Design review of the part built by this model. Coordinates are the model's own, in mm. A direction names the side the tool comes from. Round coordinates to 2 decimals unless told otherwise and drop trailing zeros. Write each loop counter-clockwise with the first axis right and the second up, starting at its lowest first coordinate (ties: lowest second). Pieces come first, ordered by that corner, then holes. Notation, with made-up numbers: (69.5, -7) - (105.5, -7) arc R28 ccw to (105.5, 28) - close; hole circle Ø5 at (27, 11.25). An arc over 180 degrees is marked (long way). Use one line per item in the form item = value.
```python
from build123d import *

# Parameters (mm, degrees)
F1_DEPTH = 50
F2_SIZE  = 1


with BuildPart() as f1:
    # F0 (on Top) → F1 (new body)
    with BuildSketch(Plane.XY):
        Polygon((-45.5, 0), (0, 0), (0, -59.5), (-4, -59.5), (-4, -62.5), (4, -62.5), (4, 4), (-14.25, 4), (-16.5, 4), (-29, 4), (-31.25, 4), (-49.5, 4), (-49.5, -62.5), (-41.5, -62.5), (-41.5, -59.5), (-45.5, -59.5), align=None)
        Polygon((-16.5, 4), (-14.25, 4), (-14.25, 6.5), (-19, 6.5), align=None)
        Polygon((-31.25, 6.5), (-31.25, 4), (-29, 4), (-26.5, 6.5), align=None)
    extrude(amount=F1_DEPTH)

    # F2
    f2_edges = [f1.edges().sort_by_distance(p)[0] for p in [
        (-19, 6.5, 25),
        (-26.5, 6.5, 25),
    ]]
    chamfer(f2_edges, length=F2_SIZE)


solid = f1.part
```
Q1. To check wall thickness, follow line 1 along X through (y, z) = (-35, 10.5); line 2 along Y through (x, z) = (-45, 25.5); line 3 along X through (y, z) = (-60, 37.5). State the ranges of each line that lie inside material, in increasing order. Write a range as from..to.
Calculated:
line_1 = -49.5..-45.5, 0..4
line_2 = -62.5..-59.5, 0..4
line_3 = -49.5..-41.5, -4..4
Q2. For P1, Ø23, axis at x = -25.5, z = 32, coming from the -Y side; P2, Ø3, axis at x = -43, z = 34, coming from the +Y side; P3, Ø1.2, axis at y = 5.5, z = 27.5, coming from the +X side, all flat-tipped, find the tip position at first contact; note any pin that passes through.
Calculated:
P1 = 0
P2 = 4
P3 = -14.25
Q3. Draft analysis for pull direction X (two halves, no side actions). For faces 6 (the flat face through (4, -30, 25)), 7 (the flat face through (-23, 0, 25)), 8 (the flat face through (-26.8, 0.3, 50)), 9 (the flat face through (-49.5, -29, 25)), state which applies: released by +X, released by -X, zero draft, split by the parting line, or undercut.
Calculated:
face_6 = released by +X
face_7 = undercut
face_8 = zero draft
face_9 = released by -X
Q4. We need section B-B on z = 11.5. Write out the cut boundary in (x, y), then the cut area to 3 significant figures.
Calculated:
outline = (-49.5, -62.5) - (-41.5, -62.5) - (-41.5, -59.5) - (-45.5, -59.5) - (-45.5, 0) - (0, 0) - (0, -59.5) - (-4, -59.5) - (-4, -62.5) - (4, -62.5) - (4, 4) - (-14.25, 4) - (-14.25, 6.5) - (-18, 6.5) - (-18.29, 5.79) - (-16.5, 4) - (-29, 4) - (-27.21, 5.79) - (-27.5, 6.5) - (-31.25, 6.5) - (-31.25, 4) - (-49.5, 4) - close
area = 755 mm2
Q5. Machinability: for faces 1 (the flat face through (-40, 4, 25)), 2 (the flat face through (0, -29, 25)), 3 (the flat face through (-41.5, -61, 25)), 4 (the flat face through (-5, 4, 25)), 5 (the flat face through (-29, 6.5, 25)), which of the approach directions +Z, -Z, +X, -X, +Y, -Y give a long, thin tool a straight path to every point of the face, cutting with its end or side? Answer none if there is none.
Calculated:
face_1 = +Z, -Z, -X, +Y
face_2 = +Z, -Z
face_3 = +Z, -Z, -Y
face_4 = +Z, -Z, +X, +Y
face_5 = +Z, -Z, +X, -X, +Y
Q6. We need section A-A on y = -38. Write out the cut boundary in (x, z), then the cut area to 3 significant figures.
Calculated:
outline = (-49.5, 0) - (-45.5, 0) - (-45.5, 50) - (-49.5, 50) - close; (0, 0) - (4, 0) - (4, 50) - (0, 50) - close
area = 400 mm2
